Part model, mm, in its own coordinate system. A direction names the side the tool comes from. Round coordinates to 2 decimals unless told otherwise and drop trailing zeros. Write each loop counter-clockwise with the first axis right and the second up, starting at its lowest first coordinate (ties: lowest second). Pieces come first, ordered by that corner, then holes.
1) Flat gauge pins, fed straight in: pin 1 (1.8 mm diameter, centred on x = -8, z = 4, fed in from +Y); pin 2 (2.5 mm diameter, centred on x = -9.4, z = 4, fed in from +Y) (3 decimals); pin 3 (1.2 mm diameter, centred on y = -2.5, z = 2, fed in from +X). Where does each tip first touch, or does it go through?
2) Saw through at C-C on y = -4.4. Write the cut outline in (x, z), and give its area (3 significant figures).
3) Pull direction X, two halves, no side cores. Call faces 1 (the flat face through (8, -4, 5)), 2 (the flat face through (11.8, -5, 4)), 3 (the cylindrical face through (8.13, -5.01, 4.28)): +X half, -X half, draft (parallel to the pull), parting line (faces both ways), or undercut.
4) Saw through at D-D on z = 5. Write the cut outline in (x, y), and give its area (3 significant figures).
5) Drill centre lines: L1, parallel to X at y = -5.4, z = 4; L2, parallel to X at y = -3.9, z = 7; L3, parallel to Y at x = 8, z = 6. Where is each one in solid material? Low to high.
6) Saw through at B-B on x = 9.4. Write the cut outline in (y, z).
7) Saw through at A-A on z = 3.5. Write the cut outline in (x, y).
8) Which spindle directions (+Z, -Z, +X, -X, +Y, -Y) get a long thin tool onto all of the face, cutting with end or side? Do faces 4 (the flat face through (5.65, -2, 4)), 5 (the flat face through (0, -4, 0)), 6 (the flat face through (-8, -4, 5)). Say none if no direction does.
```python
from build123d import *

# Parameters (mm, degrees)
EXTRUDE_1_DEPTH     = 8
CUT_EXTRUDE_1_REACH = 17.467
SKETCH_2_R          = 1.3


with BuildPart() as part:
    # Эскиз1 → Бобышка-Вытянуть1 (new body)
    with BuildSketch(Plane.XY):
        Polygon((-5.65, 0), (5.65, 0), (5.65, -4), (11.8, -4), (11.8, -6), (-11.8, -6), (-11.8, -4), (-5.65, -4), align=None)
    extrude(amount=EXTRUDE_1_DEPTH)

    # Эскиз2 → Вырез-Вытянуть1 (cut, up to next)
    with BuildSketch(Plane.XZ.offset(6), mode=Mode.PRIVATE) as cut_extrude_1_sk1:
        with Locations(Location((-9.4, 4, 0), (0, 0, 270))):
            Circle(SKETCH_2_R)
    cut_extrude_1_tool1 = extrude(cut_extrude_1_sk1.sketch, amount=-CUT_EXTRUDE_1_REACH, mode=Mode.PRIVATE) & part.part
    # Эскиз2 → Вырез-Вытянуть1 (cut, up to next)
    with BuildSketch(Plane.XZ.offset(6), mode=Mode.PRIVATE) as cut_extrude_1_sk2:
        with Locations(Location((9.4, 4, 0), (0, 0, 270))):
            Circle(SKETCH_2_R)
    cut_extrude_1_tool2 = extrude(cut_extrude_1_sk2.sketch, amount=-CUT_EXTRUDE_1_REACH, mode=Mode.PRIVATE) & part.part
    add(cut_extrude_1_tool1.solids().sort_by_distance((-9.4, -6, 4))[0], mode=Mode.SUBTRACT)
    add(cut_extrude_1_tool2.solids().sort_by_distance((9.4, -6, 4))[0], mode=Mode.SUBTRACT)


solid = part.part
```
Completed:
1. pin 1: stops at y = -4
1. pin 2: passes through
1. pin 3: stops at x = 5.65
2. outline: (-11.8, 0) - (11.8, 0) - (11.8, 8) - (-11.8, 8) - close; hole circle Ø2.6 at (-9.4, 4); hole circle Ø2.6 at (9.4, 4)
2. area: 178 mm2
3. face 1: draft
3. face 2: +X half
3. face 3: undercut
4. outline: (-11.8, -6) - (-10.23, -6) - (-10.23, -4) - (-11.8, -4) - close; (-8.57, -6) - (8.57, -6) - (8.57, -4) - (5.65, -4) - (5.65, 0) - (-5.65, 0) - (-5.65, -4) - (-8.57, -4) - close; (10.23, -6) - (11.8, -6) - (11.8, -4) - (10.23, -4) - close
4. area: 85.8 mm2
5. L1: x = -11.8 to -10.7, -8.1 to 8.1, 10.7 to 11.8
5. L2: x = -5.65 to 5.65
5. L3: y = -6 to -4
6. outline: (-6, 0) - (-4, 0) - (-4, 2.7) - (-6, 2.7) - close; (-6, 5.3) - (-4, 5.3) - (-4, 8) - (-6, 8) - close
7. outline: (-11.8, -6) - (-10.6, -6) - (-10.6, -4) - (-11.8, -4) - close; (-8.2, -6) - (8.2, -6) - (8.2, -4) - (5.65, -4) - (5.65, 0) - (-5.65, 0) - (-5.65, -4) - (-8.2, -4) - close; (10.6, -6) - (11.8, -6) - (11.8, -4) - (10.6, -4) - close
8. face 4: +Z, -Z, +X, +Y
8. face 5: -Z, +X, -X, +Y, -Y
8. face 6: +Z, -Z, -X, +Y
